Work out the finished part from the listing and answer in its coordinate system (mm). A direction names the side the tool comes from. Round coordinates to 2 decimals unless told otherwise and drop trailing zeros. Order: outer loops, then holes, each group sorted by start corner. A loop starts at its lowest first (then second) coordinate and runs counter-clockwise, first axis right, second up. Notation, with made-up numbers: (-9.5, 83.25) - (13.5, 83.25) arc R7 ccw to (13.5, 90.25) - close; hole circle Ø3 at (23, 35.5). An arc over 180 degrees is marked (long way). Use one line per item in the form item = value. Start each with the question number.
Q1. Find the intervals of material crossed by line 1 (Y direction, x = -20, z = 2.05); line 2 (X direction, y = 0.25, z = 1.5); line 3 (Y direction, x = 7, z = 0.2) (3 decimals), in increasing order. Write a range as [from, to].
Q2. Which of the six approach directions +Z, -Z, +X, -X, +Y, -Y give full straight-line access (tool end or side, diameter ignored) to faces 1 (the cylindrical face through (-49.245, -0.033, 1.521)), 2 (the flat face through (-20, 2, 3))?
Q3. The part is cut by section A-A on x = -12. Determine the outline of the cut face in (y, z).
Q4. The part is cut by section C-C on z = 1.9. Determine the outline of the cut face in (x, y).
Q5. Given P1, Ø1, axis at y = -1.5, z = 1.5, coming from the -X side, flat-ended and moving along its own axis, determine where the tip first touches the part or whether it passes through.
Q6. For a pull along X with two mould halves and no side action, classify faces 3 (the flat face through (-20, 2, 0)), 4 (the flat face through (-29, 1.483, 2)), 5 (the cylindrical face through (-57.85, -0.09, 1.48)) as +X half, -X half, draft (parallel to the pull), parting line (faces both ways), or undercut.
Q7. The part is cut by section D-D on x = 6.5. Determine the outline of the cut face in (y, z).
Q8. The part is cut by section B-B on y = 0. Determine the outline of the cut face in (x, z), plus the area to 3 significant figures.
from build123d import *

# Parameters (mm, degrees)
EXTRUDE_1_DEPTH     = 3
SKETCH_7_R          = 1.6
CUT_EXTRUDE_1_DEPTH = 3


with BuildPart() as part:
    # 草图1 → 凸台-拉伸1 (new body)
    with BuildSketch(Plane.XY):
        with BuildLine():
            Line((-53.850242828, 4), (13.149757172, 4))
            ThreePointArc((13.149757172, 4), (17.149757172, 0), (13.149757172, -4))
            Line((13.149757172, -4), (-53.850242828, -4))
            ThreePointArc((-53.850242828, -4), (-57.850242828, 0), (-53.850242828, 4))
        make_face()
    extrude(amount=EXTRUDE_1_DEPTH)

    # 草图7 → 切除-拉伸1 (cut)
    with BuildSketch(Plane.XY.offset(3)):
        with Locations((-53.850242828, 0)):
            Circle(SKETCH_7_R)
        with BuildLine():
            Line((-47.761926325, 1.483471582), (-10.194558278, 1.483471582))
            ThreePointArc((-10.194558278, 1.483471582), (-8.711086696, 0), (-10.194558278, -1.483471582))
            Line((-10.194558278, -1.483471582), (-47.761926325, -1.483471582))
            ThreePointArc((-47.761926325, -1.483471582), (-49.245397907, 0), (-47.761926325, 1.483471582))
        make_face()
        with BuildLine():
            Line((5.076512497, 1.6), (13.149757172, 1.6))
            ThreePointArc((13.149757172, 1.6), (14.744323235, 0.131753831), (13.412369906, -1.57830116))
            Line((13.412369906, -1.57830116), (5.076512497, -1.6))
            ThreePointArc((5.076512497, -1.6), (3.476512497, 0), (5.076512497, 1.6))
        make_face()
    extrude(amount=-CUT_EXTRUDE_1_DEPTH, mode=Mode.SUBTRACT)


solid = part.part
Found:
q1.line_1 = [-4, -1.48], [1.48, 4]
q1.line_2 = [-57.84, -55.43], [-52.27, -49.22], [-8.73, 3.5], [14.73, 17.14]
q1.line_3 = [-4, -1.595], [1.6, 4]
q2.face_1 = +Z, -Z
q2.face_2 = +Z, +X, -X, +Y, -Y
q3.outline = (-4, 0) - (-1.48, 0) - (-1.48, 3) - (-4, 3) - close; (1.48, 0) - (4, 0) - (4, 3) - (1.48, 3) - close
q4.outline = (-53.85, -4) - (13.15, -4) arc R4 ccw to (13.15, 4) - (-53.85, 4) arc R4 ccw to start; hole circle Ø3.2 at (-53.85, 0); hole (-47.76, -1.48) - (-10.19, -1.48) arc R1.48 ccw to (-10.19, 1.48) - (-47.76, 1.48) arc R1.48 ccw to start; hole (5.08, -1.6) - (13.41, -1.58) arc R1.6 ccw to (13.15, 1.6) - (5.08, 1.6) arc R1.6 ccw to start
q5.P1 = -57.72
q6.face_3 = draft
q6.face_4 = undercut
q6.face_5 = -X half
q7.outline = (-4, 0) - (-1.6, 0) - (-1.6, 3) - (-4, 3) - close; (1.6, 0) - (4, 0) - (4, 3) - (1.6, 3) - close
q8.outline = (-57.85, 0) - (-55.45, 0) - (-55.45, 3) - (-57.85, 3) - close; (-52.25, 0) - (-49.25, 0) - (-49.25, 3) - (-52.25, 3) - close; (-8.71, 0) - (3.48, 0) - (3.48, 3) - (-8.71, 3) - close; (14.75, 0) - (17.15, 0) - (17.15, 3) - (14.75, 3) - close
q8.area = 60.0 mm²
